from build123d import *

# Parameters (mm, degrees)
BOSS_EXTRUDE1_DEPTH = 6
FILLET1_R           = 20
SKETCH5_R           = 2.2
CUT_EXTRUDE3_DEPTH  = 10
SKETCH6_W           = 18
SKETCH6_H           = 7
CUT_EXTRUDE4_DEPTH  = 10
FILLET3_R           = 2
SKETCH9_R           = 1.7
CUT_EXTRUDE7_DEPTH  = 70
SKETCH14_R          = 10
CUT_EXTRUDE10_DEPTH = 43
SKETCH15_W          = 10
SKETCH15_H          = 4
CUT_EXTRUDE11_DEPTH = 10
SKETCH16_R          = 1.65
SKETCH16_R_2        = 17
CUT_EXTRUDE12_DEPTH = 10
SKETCH19_R          = 2.2
CUT_EXTRUDE14_DEPTH = 10
SKETCH23_R          = 2.15
CUT_EXTRUDE15_DEPTH = 10


with BuildPart() as part:
    # Sketch1 → Boss-Extrude1 (new body)
    with BuildSketch(Plane.XY):
        Polygon((80, 138.564064606), (-80, 138.564064606), (-160, 0), (-80, -138.564064606), (80, -138.564064606), (160, 0), align=None)
    extrude(amount=BOSS_EXTRUDE1_DEPTH)

    # Fillet1
    fillet1_edges = [part.edges().sort_by_distance(p)[0] for p in [
        (160, 0, 3),
        (80, -138.564064606, 3),
        (-80, -138.564064606, 3),
        (-160, 0, 3),
        (-80, 138.564064606, 3),
        (80, 138.564064606, 3),
    ]]
    fillet(fillet1_edges, radius=FILLET1_R)

    # Sketch5 → Cut-Extrude3 (cut)
    with BuildSketch(Plane.XY.offset(6)):
        with Locations((-66, -113.564064606)):
            Circle(SKETCH5_R)
        with Locations((-15, -113.564064606)):
            Circle(SKETCH5_R)
        with Locations((15, -113.564064606)):
            Circle(SKETCH5_R)
        with Locations((66, -113.564064606)):
            Circle(SKETCH5_R)
        with Locations((-65.349364905, 113.939708953)):
            Circle(SKETCH5_R)
        with Locations((-90.849364905, 69.77241336)):
            Circle(SKETCH5_R)
        with Locations((-105.849364905, 43.791651246)):
            Circle(SKETCH5_R)
        with Locations((-131.349364905, -0.375644347)):
            Circle(SKETCH5_R)
        with Locations((131.349364905, -0.375644347)):
            Circle(SKETCH5_R)
        with Locations((105.849364905, 43.791651246)):
            Circle(SKETCH5_R)
        with Locations((90.849364905, 69.77241336)):
            Circle(SKETCH5_R)
        with Locations((65.349364905, 113.939708953)):
            Circle(SKETCH5_R)
    extrude(amount=-CUT_EXTRUDE3_DEPTH, mode=Mode.SUBTRACT)

    # Sketch6 → Cut-Extrude4 (cut)
    with BuildSketch(Plane.XY.offset(6)):
        with Locations((-40.5, -125.464064606)):
            Rectangle(SKETCH6_W, SKETCH6_H)
        with Locations((40.5, -125.464064606)):
            Rectangle(SKETCH6_W, SKETCH6_H)
        Polygon((-86.936156124, 107.35028979), (-95.936156124, 91.761832522), (-89.873978297, 88.261832522), (-80.873978297, 103.85028979), align=None)
        Polygon((-127.436156124, 37.202232084), (-121.373978297, 33.702232084), (-130.373978297, 18.113774815), (-136.436156124, 21.613774815), align=None)
        Polygon((136.436156124, 21.613774815), (127.436156124, 37.202232084), (121.373978297, 33.702232084), (130.373978297, 18.113774815), align=None)
        Polygon((95.936156124, 91.761832522), (89.873978297, 88.261832522), (80.873978297, 103.85028979), (86.936156124, 107.35028979), align=None)
    extrude(amount=-CUT_EXTRUDE4_DEPTH, mode=Mode.SUBTRACT)

    # Fillet3
    fillet3_edges = [part.edges().sort_by_distance(p)[0] for p in [
        (121.373978297, 33.702232084, 3),
        (127.436156124, 37.202232084, 3),
        (136.436156124, 21.613774815, 3),
        (130.373978297, 18.113774815, 3),
        (-130.373978297, 18.113774815, 3),
        (-136.436156124, 21.613774815, 3),
        (-127.436156124, 37.202232084, 3),
        (-121.373978297, 33.702232084, 3),
        (-89.873978297, 88.261832522, 3),
        (-95.936156124, 91.761832522, 3),
        (-86.936156124, 107.35028979, 3),
        (-80.873978297, 103.85028979, 3),
        (49.5, -121.964064606, 3),
        (49.5, -128.964064606, 3),
        (31.5, -128.964064606, 3),
        (31.5, -121.964064606, 3),
        (80.873978297, 103.85028979, 3),
        (86.936156124, 107.35028979, 3),
        (95.936156124, 91.761832522, 3),
        (89.873978297, 88.261832522, 3),
        (-31.5, -121.964064606, 3),
        (-31.5, -128.964064606, 3),
        (-49.5, -128.964064606, 3),
        (-49.5, -121.964064606, 3),
    ]]
    fillet(fillet3_edges, radius=FILLET3_R)

    # Sketch9 → Cut-Extrude7 (cut)
    with BuildSketch(Plane.XY.offset(6)):
        with Locations((-75.381197846, -130.564064606)):
            Circle(SKETCH9_R)
        with Locations((75.381197846, -130.564064606)):
            Circle(SKETCH9_R)
        with Locations((-75.381197846, 130.564064606)):
            Circle(SKETCH9_R)
        with Locations((-150.762395693, 0)):
            Circle(SKETCH9_R)
        with Locations((150.762395693, 0)):
            Circle(SKETCH9_R)
        with Locations((75.381197846, 130.564064606)):
            Circle(SKETCH9_R)
    extrude(amount=-CUT_EXTRUDE7_DEPTH, mode=Mode.SUBTRACT)

    # Sketch14 → Cut-Extrude10 (cut)
    with BuildSketch(Plane.XY.offset(6)):
        Circle(SKETCH14_R)
    extrude(amount=-CUT_EXTRUDE10_DEPTH, mode=Mode.SUBTRACT)

    # Sketch15 → Cut-Extrude11 (cut)
    with BuildSketch(Plane.XY.offset(6)):
        Polygon((-109.579927657, -16.669872981), (-106.115826042, -18.669872981), (-111.115826042, -27.330127019), (-114.579927657, -25.330127019), align=None)
        Polygon((-35.353430349, 111.894191624), (-40.353430349, 103.233937587), (-36.889328734, 101.233937587), (-31.889328734, 109.894191624), align=None)
        Polygon((40.353430349, 103.233937587), (36.889328734, 101.233937587), (31.889328734, 109.894191624), (35.353430349, 111.894191624), align=None)
        Polygon((114.579927657, -25.330127019), (109.579927657, -16.669872981), (106.115826042, -18.669872981), (111.115826042, -27.330127019), align=None)
        with Locations((74.226497308, -84.564064606)):
            Rectangle(SKETCH15_W, SKETCH15_H)
        with Locations((-74.226497308, -84.564064606)):
            Rectangle(SKETCH15_W, SKETCH15_H)
    extrude(amount=-CUT_EXTRUDE11_DEPTH, mode=Mode.SUBTRACT)

    # Sketch16 → Cut-Extrude12 (cut)
    with BuildSketch(Plane.XY.offset(6)):
        with Locations((15.75, 74.314064606)):
            Circle(SKETCH16_R)
        with Locations((-15.75, 74.314064606)):
            Circle(SKETCH16_R)
        with Locations((15.75, 42.814064606)):
            Circle(SKETCH16_R)
        with Locations((-15.75, 42.814064606)):
            Circle(SKETCH16_R)
        with Locations((0, 58.564064606)):
            Circle(SKETCH16_R_2)
    extrude(amount=-CUT_EXTRUDE12_DEPTH, mode=Mode.SUBTRACT)

    # Sketch19 → Cut-Extrude14 (cut)
    with BuildSketch(Plane.XY.offset(6)):
        with Locations((-98.349364905, 56.782032303)):
            Circle(SKETCH19_R)
        with Locations((98.349364905, 56.782032303)):
            Circle(SKETCH19_R)
        with Locations((0, -113.564064606)):
            Circle(SKETCH19_R)
    extrude(amount=-CUT_EXTRUDE14_DEPTH, mode=Mode.SUBTRACT)

    # Sketch23 → Cut-Extrude15 (cut)
    with BuildSketch(Plane.XY.offset(6)):
        with Locations((79.176497308, -67.564064606)):
            Circle(SKETCH23_R)
        with Locations((69.276497308, -67.564064606)):
            Circle(SKETCH23_R)
        with Locations((-69.276497308, -67.564064606)):
            Circle(SKETCH23_R)
        with Locations((-79.176497308, -67.564064606)):
            Circle(SKETCH23_R)
        with Locations((-98.100444985, -34.786825749)):
            Circle(SKETCH23_R)
        with Locations((-93.150444985, -26.213174251)):
            Circle(SKETCH23_R)
        with Locations((-23.873947677, 93.777238857)):
            Circle(SKETCH23_R)
        with Locations((-18.923947677, 102.350890354)):
            Circle(SKETCH23_R)
        with Locations((18.923947677, 102.350890354)):
            Circle(SKETCH23_R)
        with Locations((23.873947677, 93.777238857)):
            Circle(SKETCH23_R)
        with Locations((93.150444985, -26.213174251)):
            Circle(SKETCH23_R)
        with Locations((98.100444985, -34.786825749)):
            Circle(SKETCH23_R)
    extrude(amount=-CUT_EXTRUDE15_DEPTH, mode=Mode.SUBTRACT)


solid = part.part
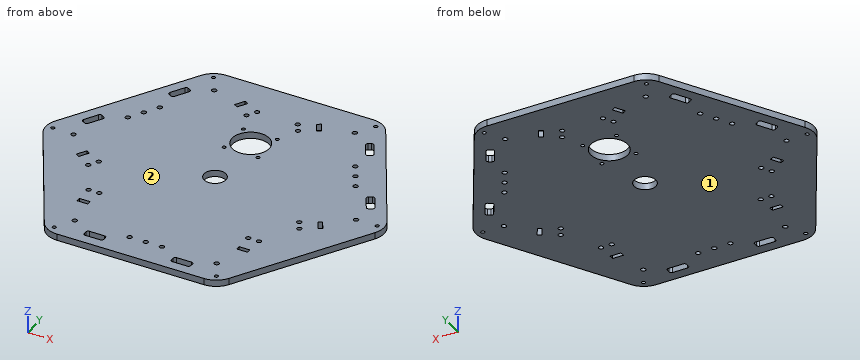
For this review, take the finished solid that the model builds, in its own axes (mm). Face numbers are marked on the shaded views. Round coordinates to 2 decimals unless told otherwise and drop trailing zeros. Put each result on its own line as item: value. Start each with the question number.
1. Insertion check: P1, Ø4, axis at x = 15, y = -113.56, coming from the +Z side; P2, Ø3, axis at y = -85, z = 2.5, coming from the +X side; P3, Ø1.2, axis at y = -84.5, z = 2, coming from the -X side. Each pin has a flat end and moves straight along its axis. Give the tip position at first contact, or say it passes through.
2. Mouldability with a two-part tool opening along Z and no side actions: class the marked faces 1 and 2 as +Z half, -Z half, draft (parallel to the pull), parting line (faces both ways), or undercut.
3. Consider section A-A on z = 2.5. State how many separate pieces and enclosed holes the cut face has, plus the area to 3 significant figures.
4. For probe 1 along Y at (x, z) = (-44, 1.25); probe 2 along X at (y, z) = (26, 5.5); probe 3 along Y at (x, z) = (15, 4.7), list the stretches that pass through material, from the lowest coordinate up. Write a range as [from, to].
Result sheet:
1. P1: through
1. P2: x = 111.79
1. P3: x = -111.56
2. face 1: -Z half
2. face 2: +Z half
3. separate pieces: 1
3. enclosed holes: 51
3. area: 63,700 mm^2
4. probe 1: [-138.56, -128.96], [-121.96, 138.56]
4. probe 2: [-144.99, -133.9], [-125.82, 125.82], [133.9, 144.99]
4. probe 3: [-138.56, -115.76], [-111.36, 41.34], [44.28, 50.56], [66.56, 72.84], [75.78, 138.56]
